```python
from build123d import *

# Parameters (mm, degrees)
SKETCH1_W           = 82.55
SKETCH1_H           = 101.6
BOSS_EXTRUDE1_DEPTH = 3.175
SKETCH2_R           = 3.175
SKETCH2_R_2         = 4.2164
CUT_EXTRUDE1_DEPTH  = 66.761600688
FILLET1_R           = 2.54


with BuildPart() as part:
    # Sketch1 → Boss-Extrude1 (new, symmetric)
    with BuildSketch(Plane.XY):
        Rectangle(SKETCH1_W, SKETCH1_H)
    extrude(amount=BOSS_EXTRUDE1_DEPTH, both=True)

    # Sketch2 → Cut-Extrude1 (cut, through all)
    with BuildSketch(Plane.XY.offset(3.175)):
        with Locations((-19.685, 31.75)):
            Circle(SKETCH2_R)
        with Locations((28.575, -31.75)):
            Circle(SKETCH2_R_2)
        with Locations((-28.575, -31.75)):
            Circle(SKETCH2_R_2)
        with Locations((28.575, 31.75)):
            Circle(SKETCH2_R)
    extrude(amount=-CUT_EXTRUDE1_DEPTH, mode=Mode.SUBTRACT)

    # Fillet1
    fillet1_edges = [part.edges().sort_by_distance(p)[0] for p in [
        (41.275, -50.8, 0),
        (-41.275, -50.8, 0),
        (-41.275, 50.8, 0),
        (41.275, 50.8, 0),
    ]]
    fillet(fillet1_edges, radius=FILLET1_R)


solid = part.part
```
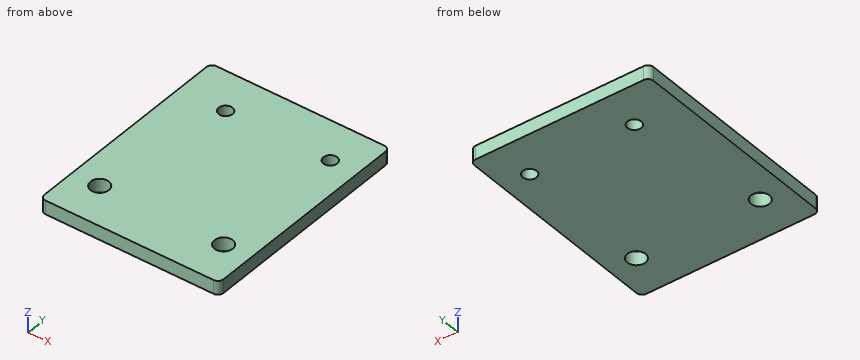
Geometry check sheet. Reference: the model listing, model coordinates, mm. Coordinates: 2 decimals unless noted, no trailing zeros. Loops run counter-clockwise (first coordinate to the right, second up) from the corner with the lowest first, then second, coordinate; pieces in that order, holes last. Notation, with made-up numbers: (-18, 63.25) -> (14, 63.25) arc R6 ccw to (14, 68.25) -> close; hole circle Ø4 at (39, 53). An arc over 180 degrees is marked (long way). Put each result on its own line as item: value.
1) Thickness scan on line 1 (Y direction, x = 26, z = 0.25); line 2 (Y direction, x = 31, z = 1.5); line 3 (X direction, y = 29, z = -2.25) (3 decimals). Record the ranges inside material, lowest first.
Result set:
line 1: y = -50.8 to -35.09, -28.41 to 29.89, 33.61 to 50.8
line 2: y = -50.8 to -35.2, -28.3 to 29.7, 33.8 to 50.8
line 3: x = -41.275 to -21.272, -18.098 to 26.988, 30.162 to 41.275
2) Cross-section at C-C on y = 31.75. Record the boundary of the cut face in (x, z) (3 decimals).
Result set:
outline: (-41.275, -3.175) -> (-22.86, -3.175) -> (-22.86, 3.175) -> (-41.275, 3.175) -> close; (-16.51, -3.175) -> (25.4, -3.175) -> (25.4, 3.175) -> (-16.51, 3.175) -> close; (31.75, -3.175) -> (41.275, -3.175) -> (41.275, 3.175) -> (31.75, 3.175) -> close
3) Cross-section at B-B on z = -0.75. Record the boundary of the cut face in (x, y) (3 decimals), plus the area to 3 significant figures.
Result set:
outline: (-41.275, -48.26) arc R2.54 ccw to (-38.735, -50.8) -> (38.735, -50.8) arc R2.54 ccw to (41.275, -48.26) -> (41.275, 48.26) arc R2.54 ccw to (38.735, 50.8) -> (-38.735, 50.8) arc R2.54 ccw to (-41.275, 48.26) -> close; hole circle Ø8.433 at (-28.575, -31.75); hole circle Ø6.35 at (-19.685, 31.75); hole circle Ø8.433 at (28.575, -31.75); hole circle Ø6.35 at (28.575, 31.75)
area: 8,210 mm^2
4) Cross-section at A-A on y = -31.75. Record the boundary of the cut face in (x, z) (3 decimals).
Result set:
outline: (-41.275, -3.175) -> (-32.791, -3.175) -> (-32.791, 3.175) -> (-41.275, 3.175) -> close; (-24.359, -3.175) -> (24.359, -3.175) -> (24.359, 3.175) -> (-24.359, 3.175) -> close; (32.791, -3.175) -> (41.275, -3.175) -> (41.275, 3.175) -> (32.791, 3.175) -> close
